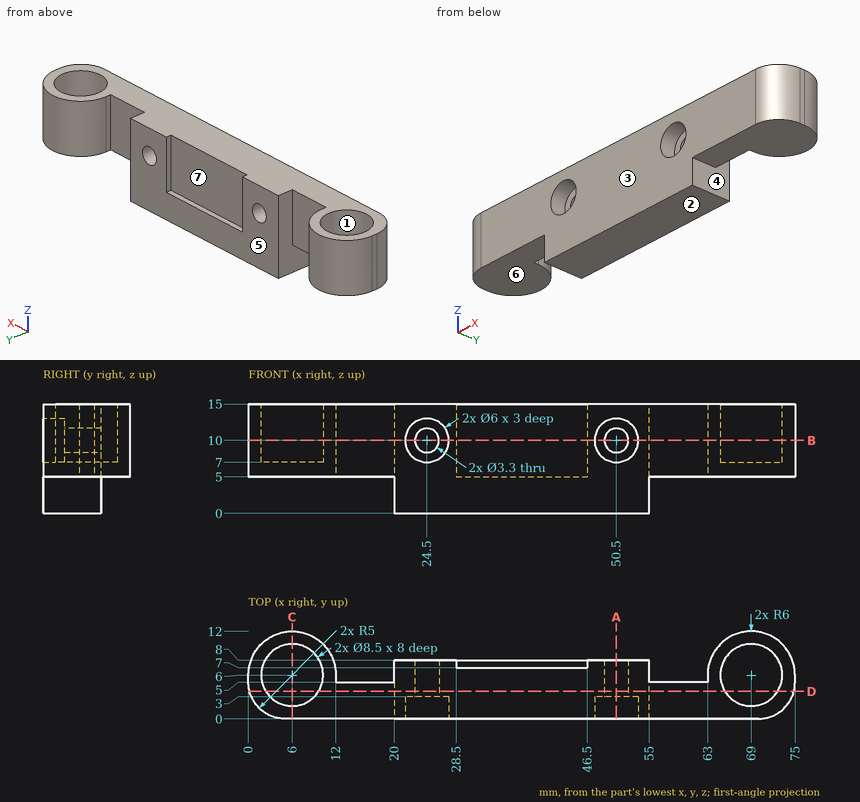
Here's the drawing with two shaded views (mm, measured from the low corner). I have some questions. A direction names the side the tool comes from. Give positions to 0.01 mm unless a question says otherwise; leave off trailing zeros. Write each loop counter-clockwise with the first axis right and the second up, starting at its lowest first coordinate (ties: lowest second). Pieces come first, ordered by that corner, then holes. Notation, with made-up numbers: (11, -3.5) - (58, -3.5) arc R16 ccw to (58, 22.5) - close; hole circle Ø8 at (58.5, -10). An arc over 180 degrees is marked (long way). Write item = value, one per line. Start each with the question number.
1. Imagine slicing it at D-D (y = 3.75). Please give me the cut outline in (x, z).
2. Imagine slicing it at B-B (z = 10). Count the separate pieces of the cut face and the enclosed holes in it, and give its area (3 significant figures).
3. Imagine slicing it at C-C (x = 6). Please give me the cut outline in (y, z).
4. Imagine slicing it at A-A (x = 50.5). Please give me the cut outline in (y, z), and give its area (3 significant figures).
5. Please list where these lines run through material, in increasing order: line 1 (X direction, y = 4.25, z = 12.5); line 2 (X direction, y = 4.1, z = 10); line 3 (Y direction, x = 6, z = 9).
6. Thinking about a two-plate mould opening in Y: for the marked faces 1, 2 and 3, which applies, released by +Y, released by -Y, zero draft, split by the parting line, or undercut?
7. On a 3-axis mill with a long thin cutter (end or side, diameter ignored), from which of +Z, -Z, +X, -X, +Y, -Y can I reach the whole of each face in a straight line? I mean the marked faces 4, 5, 6 and 7. Say none if no direction works.
8. For pin 1 (5.5 mm diameter, centred on x = 24.5, z = 10, fed in from -Y); pin 2 (5 mm diameter, centred on x = 24, z = 9.5, fed in from -Y); pin 3 (0.8 mm diameter, centred on x = 41, y = 7.5, fed in from +Z); pin 4 (4 mm diameter, centred on x = 65, y = 6.5, fed in from -Z), each with a flat end and sliding along its axis, tell me the tip position at first contact or that it passes through.
Worked answers:
q1.outline = (0.16, 5) - (20, 5) - (20, 0) - (55, 0) - (55, 5) - (74.84, 5) - (74.84, 15) - (72.61, 15) - (72.61, 7) - (65.39, 7) - (65.39, 15) - (9.61, 15) - (9.61, 7) - (2.39, 7) - (2.39, 15) - (0.16, 15) - close; hole circle Ø3.3 at (24.5, 10); hole circle Ø3.3 at (50.5, 10)
q2.separate_pieces = 3
q2.enclosed_holes = 2
q2.area = 406 mm2
q3.outline = (0, 5) - (12, 5) - (12, 15) - (10.25, 15) - (10.25, 7) - (1.75, 7) - (1.75, 15) - (0, 15) - close
q4.outline = (0, 0) - (8, 0) - (8, 8.35) - (3, 8.35) - (3, 7) - (0, 7) - close; (0, 13) - (3, 13) - (3, 11.65) - (8, 11.65) - (8, 15) - (0, 15) - close
q4.area = 85.5 mm2
q5.line_1 = 0.06 to 2.13, 9.87 to 65.13, 72.87 to 74.94
q5.line_2 = 0.08 to 2.2, 9.8 to 22.85, 26.15 to 48.85, 52.15 to 65.2, 72.8 to 74.92
q5.line_3 = 0 to 1.75, 10.25 to 12
q6.face_1 = undercut
q6.face_2 = zero draft
q6.face_3 = released by -Y
q7.face_4 = -Z, +Y
q7.face_5 = +Z, -Z, +Y
q7.face_6 = -Z, -X, +Y, -Y
q7.face_7 = +Z, +Y
q8.pin_1 = 3
q8.pin_2 = 0
q8.pin_3 = 5
q8.pin_4 = 5
